Source: CAD feature listing. Evaluate the final solid. Frame: model axes, mm. A direction names the side the tool comes from. Round coordinates to 2 decimals unless told otherwise and drop trailing zeros. Loops run counter-clockwise (first coordinate to the right, second up) from the corner with the lowest first, then second, coordinate; pieces in that order, holes last. Notation, with made-up numbers: (-2.75, 35.5) - (26.25, 35.5) arc R21 cw to (26.25, 64.5) - close; hole circle Ø9 at (61, 72). An arc over 180 degrees is marked (long way). Write item = value, one per line. Start each with the question number.
from build123d import *

# Parameters (mm, degrees)
SKIZZE1_W                                            = 42
SKIZZE1_H                                            = 50
AUFSATZ_LINEAR_AUSTRAGEN1_DEPTH                      = 7
STIRNSENKUNG_F_R_M4_ZYLINDERSCHRAUBE_MIT_D           = 4.5
STIRNSENKUNG_F_R_M4_ZYLINDERSCHRAUBE_MIT_CBORE_D     = 8
STIRNSENKUNG_F_R_M4_ZYLINDERSCHRAUBE_MIT_CBORE_DEPTH = 4.4
AUFSATZ_LINEAR_AUSTRAGEN2_DEPTH                      = 42
VERRUNDUNG1_R                                        = 0.8
SCHNITT_LINEAR_AUSTRAGEN1_DEPTH                      = 14
VERRUNDUNG2_R                                        = 5
VERRUNDUNG3_R                                        = 1.2
STIRNSENKUNG_F_R_M3_ZYLINDERSCHRAUBE_MIT_D           = 3.4
STIRNSENKUNG_F_R_M3_ZYLINDERSCHRAUBE_MIT_CBORE_D     = 6.5
STIRNSENKUNG_F_R_M3_ZYLINDERSCHRAUBE_MIT_CBORE_DEPTH = 3.4


with BuildPart() as part:
    # Skizze1 → Aufsatz-Linear austragen1 (new body)
    with BuildSketch(Plane.XY):
        Rectangle(SKIZZE1_W, SKIZZE1_H)
    extrude(amount=AUFSATZ_LINEAR_AUSTRAGEN1_DEPTH)

    # Stirnsenkung für M4 Zylinderschraube mit Innensechskant1 (through all)
    with Locations(Plane.XY.offset(7)):
        with Locations((-1.5, 17.5), (11.5, 17.5), (11.5, -17.5), (-1.5, -17.5)):
            CounterBoreHole(STIRNSENKUNG_F_R_M4_ZYLINDERSCHRAUBE_MIT_D / 2, STIRNSENKUNG_F_R_M4_ZYLINDERSCHRAUBE_MIT_CBORE_D / 2, STIRNSENKUNG_F_R_M4_ZYLINDERSCHRAUBE_MIT_CBORE_DEPTH)

    # Skizze4 → Aufsatz-Linear austragen2 (add, through all)
    with BuildSketch(Plane(origin=(21, 0, 0), x_dir=(0, 0, -1), z_dir=(1, 0, 0))):
        Polygon((-7, 2.5), (-13, 5), (-13, -5), (-7, -2.5), align=None)
    extrude(amount=-AUFSATZ_LINEAR_AUSTRAGEN2_DEPTH)

    # Verrundung1
    verrundung1_edges = [part.edges().sort_by_distance(p)[0] for p in [
        (0, 2.5, 7),
        (0, -2.5, 7),
    ]]
    fillet(verrundung1_edges, radius=VERRUNDUNG1_R)

    # Skizze5 → Schnitt-Linear austragen1 (cut, through all)
    with BuildSketch(Plane(origin=(0, 0, 0), x_dir=(-1, 0, 0), z_dir=(0, 0, -1))):
        Polygon((-21, 25), (-21, 15), (-16, 25), align=None)
        Polygon((21, 25), (16, 25), (21, 15), align=None)
        Polygon((-21, -15), (-21, -25), (-16, -25), align=None)
        Polygon((16, -25), (21, -25), (21, -15), align=None)
    extrude(amount=-SCHNITT_LINEAR_AUSTRAGEN1_DEPTH, mode=Mode.SUBTRACT)

    # Verrundung2
    verrundung2_edges = [part.edges().sort_by_distance(p)[0] for p in [
        (16, 25, 3.5),
        (21, 15, 3.5),
        (-21, 15, 3.5),
        (-16, 25, 3.5),
        (21, -15, 3.5),
        (16, -25, 3.5),
        (-16, -25, 3.5),
        (-21, -15, 3.5),
    ]]
    fillet(verrundung2_edges, radius=VERRUNDUNG2_R)

    # Verrundung3
    verrundung3_edges = [part.edges().sort_by_distance(p)[0] for p in [
        (0, -5, 13),
        (0, 5, 13),
    ]]
    fillet(verrundung3_edges, radius=VERRUNDUNG3_R)

    # Stirnsenkung für M3 Zylinderschraube mit Innensechskant1 (through all)
    with Locations(Plane(origin=(0, 0, 0), x_dir=(-1, 0, 0), z_dir=(0, 0, -1))):
        with Locations((17, 0)):
            CounterBoreHole(STIRNSENKUNG_F_R_M3_ZYLINDERSCHRAUBE_MIT_D / 2, STIRNSENKUNG_F_R_M3_ZYLINDERSCHRAUBE_MIT_CBORE_D / 2, STIRNSENKUNG_F_R_M3_ZYLINDERSCHRAUBE_MIT_CBORE_DEPTH)


solid = part.part
(1) Cut plane A-A (x = -1.5). Output: boundary loops of the cut face in (y, z).
(2) Mould query, pull axis Y, two halves, no side actions, for faces 1 (the face through (21, 0, 5)), 2 (the face through (-1.012, -19.696, 1.282)), 3 (the face through (0, -25, 3)). Classes: +Y half, -Y half, draft (parallel to the pull), parting line (faces both ways), or undercut.
(3) Cut plane D-D (y = 0). Output: boundary loops of the cut face in (x, z), and give its area (3 significant figures).
(4) Material intervals for line 1 along Y through (x, z) = (-1.5, 1.15); line 2 along Y through (x, z) = (11.5, 4.1); line 3 along Z through (x, y) = (15.5, 3), sorted ascending. Write a range as from..to.
(5) Access query for faces 4 (the face through (-0.29, -4.21, 12.45)), 5 (the face through (-18.4, -1.4, 3.4)), 6 (the face through (0, 25, 3)), 7 (the face through (-2.021, 21.466, 4.831)), 8 (the face through (0.294, 3.625, 9.7)). Directions: +Z, -Z, +X, -X, +Y, -Y. A direction counts if a zero-diameter tool reaches every point of the face in a straight line with its end or side. Return the directions, or none.
(6) Cut plane B-B (y = -17.5). Output: boundary loops of the cut face in (x, z), and give its area (3 significant figures).
(7) Pin query (flat end, axial travel): P1, Ø6.5, axis at x = -1.5, y = -17.5, coming from the +Z side; P2, Ø6.5, axis at x = 1.5, y = -13.5, coming from the +Z side; P3, Ø4, axis at x = -17, y = 0, coming from the -Z side. Return the tip coordinate at first contact, or that it passes through.
(8) Cut plane C-C (z = 2). Output: boundary loops of the cut face in (x, y).
Solution:
q1.outline = (-25, 0) - (-19.75, 0) - (-19.75, 2.6) - (-21.5, 2.6) - (-21.5, 7) - (-25, 7) - close; (-15.25, 0) - (15.25, 0) - (15.25, 2.6) - (13.5, 2.6) - (13.5, 7) - (3.7, 7) arc R0.8 cw to (2.96, 8.11) - (4.31, 11.34) arc R1.2 ccw to (3.2, 13) - (-3.2, 13) arc R1.2 ccw to (-4.31, 11.34) - (-2.96, 8.11) arc R0.8 cw to (-3.7, 7) - (-13.5, 7) - (-13.5, 2.6) - (-15.25, 2.6) - close; (19.75, 0) - (25, 0) - (25, 7) - (21.5, 7) - (21.5, 2.6) - (19.75, 2.6) - close
q2.face_1 = draft
q2.face_2 = undercut
q2.face_3 = -Y half
q3.outline = (-21, 0) - (-20.25, 0) - (-20.25, 3.4) - (-18.7, 3.4) - (-18.7, 13) - (-21, 13) - close; (-15.3, 3.4) - (-13.75, 3.4) - (-13.75, 0) - (21, 0) - (21, 13) - (-15.3, 13) - close
q3.area = 491 mm^2
q4.line_1 = -25..-19.75, -15.25..15.25, 19.75..25
q4.line_2 = -25..-21.5, -13.5..13.5, 21.5..25
q4.line_3 = 0..7.41, 8.2..13
q5.face_4 = +X, -X, -Y
q5.face_5 = -Z
q5.face_6 = +Z, -Z, +X, -X, +Y
q5.face_7 = +Z
q5.face_8 = +X, -X, +Y
q6.outline = (-19.75, 0) - (-3.75, 0) - (-3.75, 2.6) - (-5.5, 2.6) - (-5.5, 7) - (-19.75, 7) - close; (0.75, 0) - (9.25, 0) - (9.25, 2.6) - (7.5, 2.6) - (7.5, 7) - (2.5, 7) - (2.5, 2.6) - (0.75, 2.6) - close; (13.75, 0) - (19.75, 0) - (19.75, 7) - (15.5, 7) - (15.5, 2.6) - (13.75, 2.6) - close
q6.area = 183 mm^2
q7.P1 = 2.6
q7.P2 = 7
q7.P3 = 3.4
q8.outline = (-21, -13.82) arc R5 ccw to (-20.47, -16.06) - (-17.38, -22.24) arc R5 ccw to (-12.91, -25) - (12.91, -25) arc R5 ccw to (17.38, -22.24) - (20.47, -16.06) arc R5 ccw to (21, -13.82) - (21, 13.82) arc R5 ccw to (20.47, 16.06) - (17.38, 22.24) arc R5 ccw to (12.91, 25) - (-12.91, 25) arc R5 ccw to (-17.38, 22.24) - (-20.47, 16.06) arc R5 ccw to (-21, 13.82) - close; hole circle Ø6.5 at (-17, 0); hole circle Ø4.5 at (-1.5, -17.5); hole circle Ø4.5 at (-1.5, 17.5); hole circle Ø4.5 at (11.5, -17.5); hole circle Ø4.5 at (11.5, 17.5)
